from build123d import *

# Parameters (mm, degrees)
EXTRUDE_2_DEPTH = 25.4
EXTRUDE_START   = 2.54
EXTRUDE_4_DEPTH = 2.54
SKETCH_4_R      = 2.623574207
EXTRUDE_5_DEPTH = 12.7


with BuildPart() as part:
    # 草图2 → 凸台-拉伸2 (new body)
    with BuildSketch(Plane(origin=(0, 0, 0), x_dir=(1, 0, 0), z_dir=(0, 1, 0))):
        with BuildLine():
            Line((27.862923991, 48.26), (25.533011104, 48.26))
            Line((25.533011104, 48.26), (19.005421019, 35.922187738))
            ThreePointArc((19.005421019, 35.922187738), (0.578570421, 40.635881389), (-17.97500995, 36.448712149))
            Line((-17.97500995, 36.448712149), (-24.735061671, 48.26))
            Line((-24.735061671, 48.26), (-27.862923991, 48.26))
            Line((-27.862923991, 48.26), (-55.725847982, 0))
            Line((-55.725847982, 0), (-54.259378298, -2.54))
            Line((-54.259378298, -2.54), (-40.560547334, -2.54))
            ThreePointArc((-40.560547334, -2.54), (-35.350417354, -20.048880091), (-22.997765154, -33.50690075))
            Line((-22.997765154, -33.50690075), (-28.222727801, -42.556801521))
            Line((-28.222727801, -42.556801521), (-29.689197484, -45.096801521))
            Line((-29.689197484, -45.096801521), (-27.862923991, -48.26))
            Line((-27.862923991, -48.26), (27.862923991, -48.26))
            Line((27.862923991, -48.26), (29.124677573, -46.07457869))
            Line((29.124677573, -46.07457869), (22.183228773, -34.051636689))
            ThreePointArc((22.183228773, -34.051636689), (34.920508786, -20.78864272), (40.508274586, -3.269447975))
            Line((40.508274586, -3.269447975), (53.838231313, -3.269447975))
            Line((53.838231313, -3.269447975), (55.725847982, 0))
            Line((55.725847982, 0), (27.862923991, 48.26))
        make_face()
        with BuildLine():
            Line((-26.301774892, 45.883989559), (-18.95614877, 33.049575244))
            ThreePointArc((-18.95614877, 33.049575244), (0.620872136, 38.094940842), (20.02308022, 32.414290961))
            Line((20.02308022, 32.414290961), (26.744142761, 45.117785934))
            Line((26.744142761, 45.117785934), (53.2140556, -0.729447975))
            Line((53.2140556, -0.729447975), (38.093016495, -0.729447975))
            ThreePointArc((38.093016495, -0.729447975), (32.721218848, -19.517475172), (18.742100855, -33.171428301))
            Line((18.742100855, -33.171428301), (25.987022104, -45.72))
            Line((25.987022104, -45.72), (-27.116061926, -45.72))
            Line((-27.116061926, -45.72), (-19.587157143, -32.679554389))
            ThreePointArc((-19.587157143, -32.679554389), (-33.150269133, -18.779500963), (-38.1, 0))
            Line((-38.1, 0), (-52.792908615, 0))
            Line((-52.792908615, 0), (-26.301774892, 45.883989559))
        make_face(mode=Mode.SUBTRACT)
    extrude(amount=EXTRUDE_2_DEPTH)

    # 草图3 → 凸台-拉伸4 (add)
    with BuildSketch(Plane.XZ.offset(EXTRUDE_START)):
        with BuildLine():
            Line((22.183228773, 34.051636689), (29.124677573, 46.07457869))
            Line((29.124677573, 46.07457869), (27.862923991, 48.26))
            Line((27.862923991, 48.26), (-27.862923991, 48.26))
            Line((-27.862923991, 48.26), (-29.689197484, 45.096801521))
            Line((-29.689197484, 45.096801521), (-22.997765154, 33.50690075))
            ThreePointArc((-22.997765154, 33.50690075), (-35.350417354, 20.048880091), (-40.560547334, 2.54))
            Line((-40.560547334, 2.54), (-54.259378298, 2.54))
            Line((-54.259378298, 2.54), (-55.725847982, 0))
            Line((-55.725847982, 0), (-27.862923991, -48.26))
            Line((-27.862923991, -48.26), (-24.735061671, -48.26))
            Line((-24.735061671, -48.26), (-17.97500995, -36.448712149))
            ThreePointArc((-17.97500995, -36.448712149), (0.578570421, -40.635881389), (19.005421019, -35.922187738))
            Line((19.005421019, -35.922187738), (25.533011104, -48.26))
            Line((25.533011104, -48.26), (27.862923991, -48.26))
            Line((27.862923991, -48.26), (55.725847982, 0))
            Line((55.725847982, 0), (53.838231313, 3.269447975))
            Line((53.838231313, 3.269447975), (40.508274586, 3.269447975))
            ThreePointArc((40.508274586, 3.269447975), (34.920508786, 20.78864272), (22.183228773, 34.051636689))
        make_face()
    extrude(amount=-EXTRUDE_4_DEPTH)

    # 草图4 → 凸台-拉伸5 (add)
    with BuildSketch(Plane(origin=(0, 0, 0), x_dir=(1, 0, 0), z_dir=(0, 1, 0))):
        with Locations(Location((0, 0, 0), (0, 0, 90))):
            Circle(SKETCH_4_R)
    extrude(amount=EXTRUDE_5_DEPTH)


solid = part.part
Part model, mm, in its own coordinate system. A direction names the side the tool comes from. Round coordinates to 2 decimals unless told otherwise and drop trailing zeros. Write each loop counter-clockwise with the first axis right and the second up, starting at its lowest first coordinate (ties: lowest second). Pieces come first, ordered by that corner, then holes. Notation, with made-up numbers: M 18,-30 L 53,-30 A35 cw 53,6 Z; hole C 45.25,-28 d4. An arc over 180 degrees is marked long. Return JSON: item names as keys, results as strings. Group by question number.
(1) Saw through at B-B on x = 0. Write the cut outline in (y, z), then the cut area to 3 significant figures.
(2) Pin check, flat tips, straight feed: pin 1 Ø6 at (y, z) = (6, -22) entering from -X; pin 2 Ø5 at (y, z) = (4, 13.5) entering from -X; pin 3 Ø3 at (y, z) = (11.5, -26.5) entering from +X. Stop position of each tip, or through.
(3) Saw through at D-D on z = 41. Write the cut outline in (x, y), then the cut area to 3 significant figures.
(4) Two-plate mould, pull along Z, no slides. Class faces 1 (the face through (23.34, 12.52, -38.68)), 2 (the face through (47, 11, 3.269)), 3 (the face through (0, 12.7, 0)), 4 (the face through (0.31, 11.23, -40.64)): +Z half, -Z half, draft (parallel to the pull), parting line (faces both ways), or undercut.
(5) Drill centre lines: probe 1 along Z at (x, y) = (-27.5, 2.5) (3 decimals); probe 2 along X at (y, z) = (12, -34.5); probe 3 along Y at (x, z) = (12, 26). Where is each one in solid material? Low to high.
(6) Saw through at A-A on y = 7.75. Count the separate pieces of the cut face and the enclosed holes in it, then the cut area to 3 significant figures.
(7) Which spindle directions (+Z, -Z, +X, -X, +Y, -Y) get a long thin tool onto all of the face, cutting with end or side? Do faces 5 (the face through (-1, -2.54, 1)), 6 (the face through (22.22, 11.23, -42)), 7 (the face through (-33.014, 12.522, 19.018)), 8 (the face through (25.605, 11.234, 39.979)). Say none if no direction does.
Returned:
{
 "1": {"outline": "M -2.54,-40.64 L 25.4,-40.64 L 25.4,-38.1 L 0,-38.1 L 0,-2.62 L 12.7,-2.62 L 12.7,2.62 L 0,2.62 L 0,45.72 L 25.4,45.72 L 25.4,48.26 L -2.54,48.26 Z", "area": "421 mm²"},
 "2": {"pin 1": "x = -44.76", "pin 2": "x = -39.12", "pin 3": "x = 41.29"},
 "3": {"outline": "M -27.32,-2.54 L 26.19,-2.54 L 26.19,25.4 L 23.26,25.4 L 23.26,0 L -24.39,0 L -24.39,25.4 L -27.32,25.4 Z", "area": "285 mm²"},
 "4": {"face 1": "undercut", "face 2": "+Z half", "face 3": "undercut", "face 4": "-Z half"},
 "5": {"probe 1": "-48.26 to -43.809, 26.37 to 29.923, 41.305 to 48.26", "probe 2": "-35.81 to -32.87, -19.79 to -16.17, 16.17 to 21.13, 32.87 to 35.81", "probe 3": "-2.54 to 0"},
 "6": {"separate pieces": "2", "enclosed holes": "1", "area": "968 mm²"},
 "7": {"face 5": "+Z, -Z, +X, -X, -Y", "face 6": "-Z, +Y, -Y", "face 7": "+Y", "face 8": "+X, +Y, -Y"}
}
